Part model, mm, in its own coordinate system. A direction names the side the tool comes from. Give positions to 0.01 mm unless a question says otherwise; leave off trailing zeros. Write each loop counter-clockwise with the first axis right and the second up, starting at its lowest first coordinate (ties: lowest second). Pieces come first, ordered by that corner, then holes. Notation, with made-up numbers: M 40,80 L 64,80 A29 cw 64,112 Z; hole C -21,6 d4. An arc over 180 degrees is marked long. Use CSV: the item, a comma, the result in double quotes. Start each with the question number.
Item 1: Cut at D-D (z = -157). List the corners of the cut face in (x, y).
Item 2: Which spindle directions (+Z, -Z, +X, -X, +Y, -Y) get a long thin tool onto all of the face, cutting with end or side? Do faces 1 (the flat face through (0, 31, -120)), 2 (the cylindrical face through (8.632, 14.777, -245.231)). Say none if no direction does.
Item 3: Cut at A-A (x = 27). List the corners of the cut face in (y, z).
Item 4: Pin check, flat tips, straight feed: pin 1 (5 mm diameter, centred on y = 6.35, z = -73.46, fed in from -X); pin 2 (5.5 mm diameter, centred on x = 9.96, y = 12.7, fed in from -Z); pin 3 (14.5 mm diameter, centred on y = 31.75, z = -129.032, fed in from +X). Stop position of each tip, or through.
Item 5: Mould opens along Y. For faces 3 (the flat face through (-2, 63.5, -123)), 4 (the cylindrical face through (-1.352, 57.01, -44.885)), 5 (the cylindrical face through (-1.06, 31.31, 0.96)), 6 (the cylindrical face through (-1.352, 7.304, -76.485)) say: released by +Y, released by -Y, zero draft, split by the parting line, or undercut.
Item 6: Drill centre lines: line 1 (Z direction, x = 45.5, y = 40.5); line 2 (X direction, y = 37, z = -144); line 3 (Z direction, x = -1, y = 31). Where is each one in solid material? Low to high. Write a range as [from, to].
Item 7: Cut at B-B (x = 10). List the corners of the cut face in (y, z), then the cut area to 3 significant figures.
Item 8: Cut at C-C (y = 6.35). Count the separate pieces of the cut face and the enclosed holes in it, then the cut area to 3 significant figures.
from build123d import *

# Parameters (mm, degrees)
BASE_FLANGE1_DEPTH = 63.5
SKETCH8_R          = 2.4638
CUT_EXTRUDE2_DEPTH = 263.252824078
SKETCH9_R          = 3.175
CUT_EXTRUDE3_DEPTH = 6.35
SKETCH10_R         = 6.35
SKETCH10_R_2       = 1.7
CUT_EXTRUDE4_DEPTH = 6.35


# Sheet-metal steps are written as plain solids
with BuildPart() as part:
    # Sketch1 → Base-Flange1 (new body)
    with BuildSketch(Plane(origin=(0, 0, 0), x_dir=(1, 0, 0), z_dir=(0, 1, 0))):
        with BuildLine():
            Line((50.8, 0), (3.175, 0))
            ThreePointArc((3.175, 0), (0.92993597, 0.92993597), (0, 3.175))
            Line((0, 3.175), (0, 240.665))
            ThreePointArc((0, 240.665), (0.92993597, 242.91006403), (3.175, 243.84))
            Line((3.175, 243.84), (50.8, 243.84))
            Line((50.8, 243.84), (50.8, 246.5832))
            Line((50.8, 246.5832), (3.175, 246.5832))
            ThreePointArc((3.175, 246.5832), (-1.009799352, 244.849799352), (-2.7432, 240.665))
            Line((-2.7432, 240.665), (-2.7432, 3.175))
            ThreePointArc((-2.7432, 3.175), (-1.009799352, -1.009799352), (3.175, -2.7432))
            Line((3.175, -2.7432), (50.8, -2.7432))
            Line((50.8, -2.7432), (50.8, 0))
        make_face()
    extrude(amount=BASE_FLANGE1_DEPTH)

    # Sketch8 → Cut-Extrude2 (cut, through all)
    with BuildSketch(Plane(origin=(0, 0, -246.5832), x_dir=(-1, 0, 0), z_dir=(0, 0, -1))):
        with Locations((-9.9568, 12.7)):
            Circle(SKETCH8_R)
        with Locations((-9.9568, 50.8)):
            Circle(SKETCH8_R)
    extrude(amount=-CUT_EXTRUDE2_DEPTH, mode=Mode.SUBTRACT)

    # Sketch9 → Cut-Extrude3 (cut)
    with BuildSketch(Plane(origin=(0, 0, 0), x_dir=(0, 0, -1), z_dir=(1, 0, 0))):
        with Locations((221.1832, 6.35)):
            Circle(SKETCH9_R)
        with Locations((195.7832, 6.35)):
            Circle(SKETCH9_R)
        with Locations((170.3832, 6.35)):
            Circle(SKETCH9_R)
        with Locations((48.0568, 6.35)):
            Circle(SKETCH9_R)
        with Locations((22.6568, 6.35)):
            Circle(SKETCH9_R)
        with Locations((73.4568, 6.35)):
            Circle(SKETCH9_R)
    cut_extrude3 = extrude(amount=-CUT_EXTRUDE3_DEPTH, mode=Mode.SUBTRACT)

    # Mirror1: Cut-Extrude3 across plane
    add(cut_extrude3.mirror(Plane.ZX.offset(31.75)), mode=Mode.SUBTRACT)

    # Sketch10 → Cut-Extrude4 (cut)
    with BuildSketch(Plane.ZY.offset(2.7432)):
        with Locations((-129.032, 31.75)):
            Circle(SKETCH10_R)
        with Locations((-121.92, 16.256)):
            Circle(SKETCH10_R_2)
        with Locations((-135.338197606, 24.003)):
            Circle(SKETCH10_R_2)
        with Locations((-135.338197606, 39.497)):
            Circle(SKETCH10_R_2)
        with Locations((-121.92, 47.244)):
            Circle(SKETCH10_R_2)
        with Locations((-108.501802394, 39.497)):
            Circle(SKETCH10_R_2)
        with Locations((-108.501802394, 24.003)):
            Circle(SKETCH10_R_2)
    extrude(amount=-CUT_EXTRUDE4_DEPTH, mode=Mode.SUBTRACT)


solid = part.part
Worked answers:
1,outline,"M -2.74,0 L 0,0 L 0,63.5 L -2.74,63.5 Z"
2,face 1,"+X, +Y, -Y"
2,face 2,"+Z, -Z"
3,outline,"M 0,-246.58 L 63.5,-246.58 L 63.5,-243.84 L 0,-243.84 Z; M 0,0 L 63.5,0 L 63.5,2.74 L 0,2.74 Z"
4,pin 1,"passes through"
4,pin 2,"stops at z = -246.58"
4,pin 3,"stops at x = 0"
5,face 3,"released by +Y"
5,face 4,"undercut"
5,face 5,"zero draft"
5,face 6,"undercut"
6,line 1,"z = [-246.58, -243.84], [0, 2.74]"
6,line 2,"x = [-2.74, 0]"
6,line 3,"z = [-244.86, -135.34], [-122.73, 1.02]"
7,outline,"M 0,-246.58 L 10.24,-246.58 L 10.24,-243.84 L 0,-243.84 Z; M 0,0 L 10.24,0 L 10.24,2.74 L 0,2.74 Z; M 15.16,-246.58 L 48.34,-246.58 L 48.34,-243.84 L 15.16,-243.84 Z; M 15.16,0 L 48.34,0 L 48.34,2.74 L 15.16,2.74 Z; M 53.26,-246.58 L 63.5,-246.58 L 63.5,-243.84 L 53.26,-243.84 Z; M 53.26,0 L 63.5,0 L 63.5,2.74 L 53.26,2.74 Z"
7,area,"294 mm^2"
8,separate pieces,"7"
8,enclosed holes,"0"
8,area,"847 mm^2"
